Part model, mm, in its own coordinate system. Give positions to 0.01 mm unless a question says otherwise; leave off trailing zeros. Write each loop counter-clockwise with the first axis right and the second up, starting at its lowest first coordinate (ties: lowest second). Pieces come first, ordered by that corner, then holes. Notation, with made-up numbers: M 66,44 L 107,44 A13 cw 107,59 Z; hole C -24,32 d10. An arc over 180 degrees is marked long. Use CSV: the item, a comma, the result in double quotes. Start each with the question number.
1. Drill centre lines: line 1 along X through (y, z) = (-1.75, 4); line 2 along X through (y, z) = (5, 13); line 3 along Z through (x, y) = (0, 10). Where is each one in solid material? Low to high. Write a range as from..to.
2. Drop flat-ended pins along their axis: pin 1 Ø7 at (x, z) = (0, 8) entering from +Y; pin 2 Ø10 at (x, y) = (109.5, -6) entering from -Z. Give the stop position or say it passes through.
3. Band-saw the part on A-A, the plane x = -116. List the corners of the cut face in (y, z).
from build123d import *

# Parameters (mm, degrees)
F0_W     = 26
F0_H     = 26
F1_DEPTH = 195.5
F4_D     = 4.5
F6_D     = 4.5
F7_W     = 20
F7_H     = 8
F8_DEPTH = 26


# Not quite as in the source:
# - a pattern or mirror of a feature is missing from the dataset's text; its kind, count and spacing are read off the source's solid


with BuildPart() as f1:
    # F0 (on Right) → F1 (new body, symmetric)
    with BuildSketch(Plane.YZ):
        with Locations((0, 13)):
            Rectangle(F0_W, F0_H)
    extrude(amount=F1_DEPTH, both=True)

    # F4 (through all)
    with Locations(Plane.XZ.offset(13)):
        with Locations((0, 8)):
            Hole(F4_D / 2)

    # F6 (through all)
    with Locations(Plane(origin=(0, 0, 0), x_dir=(1, 0, 0), z_dir=(0, 0, -1))):
        with Locations((0, -5)):
            Hole(F6_D / 2)

    # F7 (on face) → F8 (cut, through all)
    with BuildSketch(Plane.XZ.offset(13)):
        with Locations((-112.75, 4)):
            Rectangle(F7_W, F7_H)
    f8 = extrude(amount=-F8_DEPTH, mode=Mode.SUBTRACT)

    # F8_copies: F8 across plane
    add(f8.mirror(Plane(origin=(0, 0, 0), x_dir=(0, 0, 1), z_dir=(1, 0, 0))), mode=Mode.SUBTRACT)


solid = f1.part
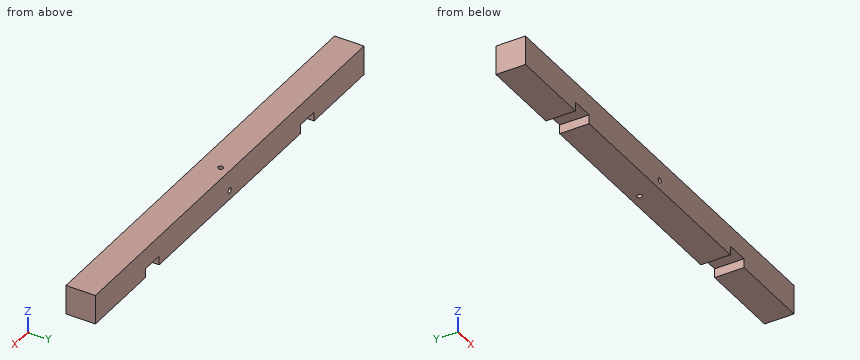
Output:
1,line 1,"x = -195.5..-122.75, -102.75..102.75, 122.75..195.5"
1,line 2,"x = -195.5..-2.25, 2.25..195.5"
1,line 3,"z = 0..5.75, 10.25..26"
2,pin 1,"stops at y = 13"
2,pin 2,"stops at z = 8"
3,outline,"M -13,8 L 13,8 L 13,26 L -13,26 Z"
